Verification items for the finished model (mm, model axes). A direction names the side the tool comes from. Round coordinates to 2 decimals unless told otherwise and drop trailing zeros. Loops run counter-clockwise (first coordinate to the right, second up) from the corner with the lowest first, then second, coordinate; pieces in that order, holes last. Notation, with made-up numbers: (-18.5, 45.5) -> (25.5, 45.5) arc R29 ccw to (25.5, 74.5) -> close; hole circle Ø10 at (-39.5, -12). An arc over 180 degrees is marked (long way). Use a Markdown table: item, result. Add a question column.
Autodesk Inventor part; units mm, degrees
ref_plane "YZ Plane" through (0, 0, 0) normal (1, 0, 0) x (0, 1, 0)
ref_plane "XZ Plane" through (0, 0, 0) normal (0, 1, 0) x (-1, 0, 0)
ref_plane "XY Plane" through (0, 0, 0) normal (0, 0, 1) x (1, 0, 0)
sketch "Sketch10" plane through (0, 0, 0) normal (0, 1, 0) x (-1, 0, 0)
  line L0 (16.6, 18.8056) -> (-16.6, 18.8056)
  line L1 (-16.6, 18.8056) -> (-16.6, -11.6944)
  line L2 (-16.6, -11.6944) -> (16.5, -11.6944)
  line L3 (16.6, 18.8056) -> (16.6, -11.6944)
  line L4 (16.6, 18.8056) -> (47.1, 18.8056) construction
  line L5 (16.6, -11.6944) -> (16.5, -11.6944)
  point P0 (0, 0)
  dimension "d53" = 33.2
  dimension "d54" = 30.5
  dimension "d55" = 90
extrude "Extrusion8" add sketch "Sketch10" against normal blind 1
sketch "Sketch11" plane through (0, -1, 0) normal (0, -1, 0) x (1, 0, 0)
  line L0 (16.6, 18.8056) -> (-16.6, 18.8056)
  line L1 (-16.6, 18.8056) -> (-15.6, 18.8056)
  line L2 (-15.6, 18.8056) -> (-15.6, 17.8056)
  line L3 (-15.6, 17.8056) -> (15.6, 17.8056)
  line L4 (15.6, 17.8056) -> (15.6, -10.6944)
  line L5 (16.6, -11.6944) -> (16.6, 18.8056)
  line L6 (15.6, -10.6944) -> (-15.6, -10.6944)
  line L7 (-15.6, -10.6944) -> (-15.6, 17.8056)
  line L8 (-16.6, -11.6944) -> (16.6, -11.6944)
  line L9 (16.6, -11.6944) -> (16.6, 18.8056)
  line L10 (16.6, 18.8056) -> (-16.6, 18.8056)
  line L11 (-16.6, 18.8056) -> (-16.6, -11.6944)
  point P0 (0, 0)
  dimension "d58" = 1
  dimension "d59" = 1
  dimension "d60" = 31.2
  dimension "d61" = 28.5
  dimension "d62" = 90
extrude "Extrusion9" add sketch "Sketch11" along normal blind 16
sketch "Sketch12" plane through (0, -17, 0) normal (0, -1, 0) x (1, 0, 0)
  point P0 (0, 0)
sketch "Sketch13" plane through (0, -17, 0) normal (0, -1, 0) x (1, 0, 0)
  line L0 (-16.6, -11.6944) -> (-16.6, 18.8056)
  line L1 (-16.6, 3.5556) -> (1.4, 3.5556)
  line L2 (1.4, 3.5556) -> (1.4, 21.0556)
  line L3 (1.4, 21.0556) -> (1.4, -13.9444)
  circle A0 centre (1.4, 21.0556) radius 2.1
  circle A1 centre (1.4, -13.9444) radius 2.1
  line L4 (-16.6, 18.8056) -> (16.6, 18.8056)
  line L5 (1.4, 18.8056) -> (5.4, 18.8056)
  line L6 (5.4, 18.8056) -> (5.4, 23.8056)
  line L7 (5.4, 23.8056) -> (-2.6, 23.8056)
  line L8 (-2.6, 23.8056) -> (-2.6, 18.8056)
  line L9 (16.6, -11.6944) -> (-16.6, -11.6944)
  line L10 (5.4, -11.6944) -> (5.4, -16.6944)
  line L11 (5.4, -16.6944) -> (-2.6, -16.6944)
  line L12 (-2.6, -16.6944) -> (-2.6, -11.6944)
  point P0 (0, 0)
  dimension "d65" = 18
  dimension "d66" = 17.5
  dimension "d67" = 35
  dimension "d68" = 4.2
  dimension "d69" = 4.2
  dimension "d70" = 4
  dimension "d71" = 5
  dimension "d72" = 90
  dimension "d73" = 8
  dimension "d74" = 5
extrude "Extrusion10" add sketch "Sketch13" against normal blind 10 contours L9 L10 L11 L12 | L8 L7 L6 L4
extrude "Extrusion11" add sketch "Sketch13" along normal blind 2 contours L9 L10 L11 L12 | L8 L7 L6 L4
properties part number "shell"
1) Thickness scan on line 1 (Z direction, x = 1.4, y = -14); line 2 (Z direction, x = -15, y = -9.5); line 3 (X direction, y = -1.25, z = -2). Record the ranges inside material, lowest first.
2) Release check for a two-part mould opening along X. For faces 5 (the face through (5.4, -13, -14)), 6 (the face through (0, -9, 17.806)), 7 (the face through (1, -13, -16.694)), 8 (the face through (2.529, -12.916, 19.285)) record: released by +X, released by -X, zero draft, split by the parting line, or undercut.
3) Sectioned sample at B-B on z = 20. Enter the section's corners in (x, y).
4) Sectioned sample at C-C on y = -2.25. Enter the section's corners in (x, z).
5) Go/stop test with flat-tipped pins: pin 1 (4 mm diameter, centred on x = 10, y = -2, fed in from -Z); pin 2 (2.5 mm diameter, centred on y = -10, z = 22, fed in from +X); pin 3 (5 mm diameter, centred on x = -0.5, z = 11.5, fed in from -Y). Record where each tip stops, or that it passes through.
6) Sectioned sample at A-A on x = 1.4. Enter the section's corners in (y, z).
7) Access from +Z, -Z, +X, -X, +Y, -Y to the whole of each face (thin tool, end or side, straight path). Record for faces 1 (the face through (0, -1, 4)), 2 (the face through (0, -7, 23)), 3 (the face through (-1, -17, -11)), 4 (the face through (0, -7, -16)).
8) Sectioned sample at D-D on y = -7.75. Enter the section's corners in (x, z).
Geometry results:
| question | item | result |
|---|---|---|
| 1 | line 1 | -16.69 to -16.04, -11.84 to -10.69, 17.81 to 18.96, 23.16 to 23.81 |
| 1 | line 2 | -11.69 to -10.69, 17.81 to 18.81 |
| 1 | line 3 | -16.6 to -15.6, 15.6 to 16.6 |
| 2 | face 5 | released by +X |
| 2 | face 6 | undercut |
| 2 | face 7 | zero draft |
| 2 | face 8 | undercut |
| 3 | outline | (-2.6, -19) -> (-0.42, -19) -> (-0.42, -7) -> (-2.6, -7) -> close; (3.22, -19) -> (5.4, -19) -> (5.4, -7) -> (3.22, -7) -> close |
| 4 | outline | (-16.6, -11.69) -> (16.6, -11.69) -> (16.6, 18.81) -> (-16.6, 18.81) -> close; hole (-15.6, -10.69) -> (15.6, -10.69) -> (15.6, 17.81) -> (-15.6, 17.81) -> close |
| 5 | pin 1 | z = -11.69 |
| 5 | pin 2 | x = 5.4 |
| 5 | pin 3 | y = -1 |
| 6 | outline | (-19, -16.69) -> (-7, -16.69) -> (-7, -16.04) -> (-19, -16.04) -> close; (-19, -11.84) -> (-7, -11.84) -> (-7, -11.69) -> (0, -11.69) -> (0, 18.81) -> (-7, 18.81) -> (-7, 18.96) -> (-19, 18.96) -> (-19, 18.81) -> (-17, 18.81) -> (-17, 17.81) -> (-1, 17.81) -> (-1, -10.69) -> (-17, -10.69) -> (-17, -11.69) -> (-19, -11.69) -> close; (-19, 23.16) -> (-7, 23.16) -> (-7, 23.81) -> (-19, 23.81) -> close |
| 7 | face 1 | -Y |
| 7 | face 2 | +Z, +X, -X, +Y |
| 7 | face 3 | +X, -X, -Y |
| 7 | face 4 | -Z, +X, -X, +Y |
| 8 | outline | (-16.6, -11.69) -> (-2.6, -11.69) -> (-2.6, -16.69) -> (5.4, -16.69) -> (5.4, -11.69) -> (16.6, -11.69) -> (16.6, 18.81) -> (5.4, 18.81) -> (5.4, 23.81) -> (-2.6, 23.81) -> (-2.6, 18.81) -> (-16.6, 18.81) -> close; hole (-15.6, -10.69) -> (15.6, -10.69) -> (15.6, 17.81) -> (-15.6, 17.81) -> close; hole circle Ø4.2 at (1.4, -13.94); hole circle Ø4.2 at (1.4, 21.06) |
